```python
from build123d import *

# Parameters (mm, degrees)
SKETCH1_W                    = 10
SKETCH1_H                    = 7.500039556
BASE_FLANGE1_DEPTH           = 1.5
EDGE_FLANGE1_STRIP_W         = 7.4732
EDGE_FLANGE1_STRIP_H         = 1.5
EDGE_FLANGE1_STRIP_CUT_DEPTH = 10
EDGE_FLANGE1_DEPTH           = 10
EDGE_FLANGE2_STRIP_W         = 7.4732
EDGE_FLANGE2_STRIP_H         = 1.5
EDGE_FLANGE2_STRIP_CUT_DEPTH = 10
EDGE_FLANGE2_DEPTH           = 10
EDGE_FLANGE3_STRIP_W         = 7.4732
EDGE_FLANGE3_STRIP_H         = 1.5
EDGE_FLANGE3_STRIP_CUT_DEPTH = 10
EDGE_FLANGE3_DEPTH           = 10
CUT_EXTRUDE1_REACH           = 165.692
SKETCH15_R                   = 1.25


# Sheet-metal steps are written as plain solids
with BuildPart() as part:
    # Sketch1 → Base-Flange1 (new body)
    with BuildSketch(Plane.XY):
        with Locations((-66, -195.249980222)):
            Rectangle(SKETCH1_W, SKETCH1_H)
    extrude(amount=BASE_FLANGE1_DEPTH)

    # Edge-Flange1 strip (across the edge) → Edge-Flange1 strip cut (cut)
    with BuildSketch(Plane(origin=(-61, -199, 0), x_dir=(0, 1, 0), z_dir=(-1, 0, 0))):
        with Locations((-3, -0.75)):
            Rectangle(EDGE_FLANGE1_STRIP_W, EDGE_FLANGE1_STRIP_H)
    extrude(amount=EDGE_FLANGE1_STRIP_CUT_DEPTH, mode=Mode.SUBTRACT)

    # Edge-Flange1 section (across the edge) → Edge-Flange1 (add)
    with BuildSketch(Plane(origin=(-61, -199, 0), x_dir=(0, 1, 0), z_dir=(-1, 0, 0))):
        with BuildLine():
            Line((-1.5, 0.7366), (-1.5, 73.5))
            Line((-1.5, 73.5), (0, 73.5))
            Line((0, 73.5), (0, 0.7366))
            ThreePointArc((0, 0.7366), (0.215745145, 0.215745145), (0.7366, 0))
            Line((0.7366, 0), (0.7366, -1.5))
            ThreePointArc((0.7366, -1.5), (-0.844915027, -0.844915027), (-1.5, 0.7366))
        make_face()
    extrude(amount=EDGE_FLANGE1_DEPTH)

    # Edge-Flange2 strip (across the edge) → Edge-Flange2 strip cut (cut)
    with BuildSketch(Plane(origin=(-61, -199, -73.5), x_dir=(0, 0, 1), z_dir=(-1, 0, 0))):
        with Locations((-3, -0.75)):
            Rectangle(EDGE_FLANGE2_STRIP_W, EDGE_FLANGE2_STRIP_H)
    extrude(amount=EDGE_FLANGE2_STRIP_CUT_DEPTH, mode=Mode.SUBTRACT)

    # Edge-Flange2 section (across the edge) → Edge-Flange2 (add)
    with BuildSketch(Plane(origin=(-61, -199, -73.5), x_dir=(0, 0, 1), z_dir=(-1, 0, 0))):
        with BuildLine():
            Line((-1.5, 0.7366), (-1.5, 124))
            Line((-1.5, 124), (0, 124))
            Line((0, 124), (0, 0.7366))
            ThreePointArc((0, 0.7366), (0.215745145, 0.215745145), (0.7366, 0))
            Line((0.7366, 0), (0.7366, -1.5))
            ThreePointArc((0.7366, -1.5), (-0.844915027, -0.844915027), (-1.5, 0.7366))
        make_face()
    extrude(amount=EDGE_FLANGE2_DEPTH)

    # Edge-Flange3 strip (across the edge) → Edge-Flange3 strip cut (cut)
    with BuildSketch(Plane(origin=(-61, -75, -73.5), x_dir=(0, -1, 0), z_dir=(-1, 0, 0))):
        with Locations((-3, -0.75)):
            Rectangle(EDGE_FLANGE3_STRIP_W, EDGE_FLANGE3_STRIP_H)
    extrude(amount=EDGE_FLANGE3_STRIP_CUT_DEPTH, mode=Mode.SUBTRACT)

    # Edge-Flange3 section (across the edge) → Edge-Flange3 (add)
    with BuildSketch(Plane(origin=(-61, -75, -73.5), x_dir=(0, -1, 0), z_dir=(-1, 0, 0))):
        with BuildLine():
            Line((-1.5, 0.7366), (-1.5, 28.5))
            Line((-1.5, 28.5), (0, 28.5))
            Line((0, 28.5), (0, 0.7366))
            ThreePointArc((0, 0.7366), (0.215745145, 0.215745145), (0.7366, 0))
            Line((0.7366, 0), (0.7366, -1.5))
            ThreePointArc((0.7366, -1.5), (-0.844915027, -0.844915027), (-1.5, 0.7366))
        make_face()
    extrude(amount=EDGE_FLANGE3_DEPTH)

    # Sketch15 → Cut-Extrude1 (cut, up to next)
    with BuildSketch(Plane(origin=(0, -73.5, 0), x_dir=(1, 0, 0), z_dir=(0, 1, 0)), mode=Mode.PRIVATE) as cut_extrude1_sk1:
        with Locations(Location((-66, 48, 0), (0, 0, 270))):
            Circle(SKETCH15_R)
    cut_extrude1_tool1 = extrude(cut_extrude1_sk1.sketch, amount=-CUT_EXTRUDE1_REACH, mode=Mode.PRIVATE) & part.part
    # Sketch15 → Cut-Extrude1 (cut, up to next)
    with BuildSketch(Plane(origin=(0, -73.5, 0), x_dir=(1, 0, 0), z_dir=(0, 1, 0)), mode=Mode.PRIVATE) as cut_extrude1_sk2:
        with Locations(Location((-66, 54, 0), (0, 0, 270))):
            Circle(SKETCH15_R)
    cut_extrude1_tool2 = extrude(cut_extrude1_sk2.sketch, amount=-CUT_EXTRUDE1_REACH, mode=Mode.PRIVATE) & part.part
    add(cut_extrude1_tool1.solids().sort_by_distance((-66, -73.5, -48))[0], mode=Mode.SUBTRACT)
    add(cut_extrude1_tool2.solids().sort_by_distance((-66, -73.5, -54))[0], mode=Mode.SUBTRACT)


solid = part.part
```
Read the model definition and answer for the solid it produces. Units are mm, in the model's axes. A direction names the side the tool comes from. Give positions to 0.01 mm unless a question says otherwise; leave off trailing zeros. Loops run counter-clockwise (first coordinate to the right, second up) from the corner with the lowest first, then second, coordinate; pieces in that order, holes last.
Item 1: The part is cut by section A-A (z = -54). Write down the section's boundary in (x, y), and give its area (4 significant figures).
Item 2: Each of these flat-tipped pins is pushed along its axis until it touches: pin 1 Ø5 at (x, z) = (-62, -15) entering from +Y; pin 2 Ø1.2 at (x, y) = (-64, -74) entering from +Z. Where does it stop, or does it pass through?
Item 3: The part is cut by section B-B (x = -66). Write down the section's boundary in (y, z), and give its area (3 significant figures).
Item 4: For faces 5 (the cylindrical face through (-64.946, -74.24, -53.328)), 6 (the flat face through (-66, -195, 0)), 7 (the flat face through (-66, -199, -37)), determine the directions among +Z, -Z, +X, -X, +Y, -Y from which every point of the face is accessible in a straight line to the end or side of a thin tool.
Item 5: The part is cut by section C-C (y = -178.5). Write down the section's boundary in (x, z).
Item 6: The part is cut by section D-D (z = -22.5). Write down the section's boundary in (x, y), and give its area (3 significant figures).
Item 7: Find the intervals of material crossed by line 1 along Y through (x, z) = (-62.5, -64.5); line 2 along Z through (x, y) = (-66, -74.05); line 3 along Z through (x, y) = (-66, -74.2), in increasing order.
Item 8: The mould has two halves that part along Z. Classify faces 1 (the cylindrical face through (-64.76, -74.24, -48.16)), 2 (the flat face through (-66, -138, -75)), 3 (the flat face through (-66, -200.5, -36)), 4 (the cylindrical face through (-65.93, -199.83, 0.86)): released by +Z, released by -Z, zero draft, split by the parting line, or undercut.
Taken from the geometry:
1. outline: (-71, -200.5) - (-61, -200.5) - (-61, -199) - (-71, -199) - close; (-71, -75) - (-67.25, -75) - (-67.25, -73.5) - (-71, -73.5) - close; (-64.75, -75) - (-61, -75) - (-61, -73.5) - (-64.75, -73.5) - close
1. area: 26.25 mm2
2. pin 1: stops at y = -199
2. pin 2: stops at z = -45
3. outline: (-200.5, -72.76) arc R2.24 ccw to (-198.26, -75) - (-75.74, -75) arc R2.24 ccw to (-73.5, -72.76) - (-73.5, -55.25) - (-75, -55.25) - (-75, -72.76) arc R0.74 cw to (-75.74, -73.5) - (-198.26, -73.5) arc R0.74 cw to (-199, -72.76) - (-199, -0.74) arc R0.74 cw to (-198.26, 0) - (-191.5, 0) - (-191.5, 1.5) - (-198.26, 1.5) arc R2.24 ccw to (-200.5, -0.74) - close; (-75, -52.75) - (-73.5, -52.75) - (-73.5, -49.25) - (-75, -49.25) - close; (-75, -46.75) - (-73.5, -46.75) - (-73.5, -45) - (-75, -45) - close
3. area: 347 mm2
4. face 5: +Y
4. face 6: +X, -X, +Y
4. face 7: +X, -X
5. outline: (-71, -75) - (-61, -75) - (-61, -73.5) - (-71, -73.5) - close
6. outline: (-71, -200.5) - (-61, -200.5) - (-61, -199) - (-71, -199) - close
6. area: 15.0 mm2
7. line 1: y = -200.5 to -199, -75 to -73.5
7. line 2: z = -74.23 to -55.25, -52.75 to -49.25, -46.75 to -45
7. line 3: z = -74.39 to -55.25, -52.75 to -49.25, -46.75 to -45
8. face 1: undercut
8. face 2: released by -Z
8. face 3: zero draft
8. face 4: released by +Z
